```python
from build123d import *

# Parameters (mm, degrees)
SKETCH_1_W             = 140
SKETCH_1_H             = 60
EXTRUDE_1_DEPTH        = 5
SKETCH_2_R             = 1.2
CUT_EXTRUDE_1096_DEPTH = 153.397506541
SKETCH_4_R             = 1.4
CUT_EXTRUDE_3_DEPTH    = 5
PATTERN_LINEAR_1_COUNT = 3
PATTERN_LINEAR_1_PITCH = 40
SKETCH_6_R             = 2
CUT_EXTRUDE_4_DEPTH    = 1


with BuildPart() as part:
    # Sketch 1 → Extrude 1 (new body)
    with BuildSketch(Plane(origin=(0, 0, 0), x_dir=(1, 0, 0), z_dir=(0, 1, 0))):
        with Locations((70, -30)):
            Rectangle(SKETCH_1_W, SKETCH_1_H)
    extrude(amount=EXTRUDE_1_DEPTH)

    # Sketch 2 → Cut-Extrude 1096 (cut, through all)
    with BuildSketch(Plane(origin=(0, 5, 0), x_dir=(1, 0, 0), z_dir=(0, 1, 0))):
        with Locations(Location((102, -15, 0), (0, 0, 270))):
            Circle(SKETCH_2_R)
        with Locations(Location((118, -15, 0), (0, 0, 270))):
            Circle(SKETCH_2_R)
        with Locations(Location((102, -45, 0), (0, 0, 90))):
            Circle(SKETCH_2_R)
        with Locations(Location((118, -45, 0), (0, 0, 90))):
            Circle(SKETCH_2_R)
        with BuildLine():
            Line((100, -26.05), (100, -36.95))
            Line((100, -36.95), (104.2, -36.95))
            Line((104.2, -36.95), (104.2, -29.381860214))
            ThreePointArc((104.2, -29.381860214), (110, -31.5), (115.8, -29.381860214))
            Line((115.8, -29.381860214), (115.8, -36.95))
            Line((115.8, -36.95), (120, -36.95))
            Line((120, -36.95), (120, -26.05))
            Line((120, -26.05), (118.270278109, -26.05))
            ThreePointArc((118.270278109, -26.05), (110, -13.5), (101.729721891, -26.05))
            Line((101.729721891, -26.05), (100, -26.05))
        make_face()
    cut_extrude_1096 = extrude(amount=-CUT_EXTRUDE_1096_DEPTH, mode=Mode.SUBTRACT)

    # Sketch 4 → Cut-Extrude 3 (cut)
    with BuildSketch(Plane.ZY):
        with Locations((30, 2.5)):
            Circle(SKETCH_4_R)
        with Locations((8, 2.5)):
            Circle(SKETCH_4_R)
        with Locations((52, 2.5)):
            Circle(SKETCH_4_R)
    cut_extrude_3 = extrude(amount=-CUT_EXTRUDE_3_DEPTH, mode=Mode.SUBTRACT)

    # Mirror 1: Cut-Extrude 3 across plane
    add(cut_extrude_3.mirror(Plane(origin=(70, 0, 0), x_dir=(0, 0, 1), z_dir=(1, 0, 0))), mode=Mode.SUBTRACT)

    # Pattern Linear 1: Cut-Extrude 1096 ×3
    with Locations(*[(-i * PATTERN_LINEAR_1_PITCH, 0, 0) for i in range(1, PATTERN_LINEAR_1_COUNT)]):
        add(cut_extrude_1096, mode=Mode.SUBTRACT)

    # Sketch 6 → Cut-Extrude 4 (cut)
    with BuildSketch(Plane.XZ):
        with Locations(Location((22, 45, 0), (0, 0, 270))):
            Circle(SKETCH_6_R)
        with Locations(Location((38, 45, 0), (0, 0, 270))):
            Circle(SKETCH_6_R)
        with Locations(Location((62, 45, 0), (0, 0, 270))):
            Circle(SKETCH_6_R)
        with Locations(Location((78, 45, 0), (0, 0, 270))):
            Circle(SKETCH_6_R)
        with Locations(Location((102, 45, 0), (0, 0, 270))):
            Circle(SKETCH_6_R)
        with Locations(Location((118, 45, 0), (0, 0, 270))):
            Circle(SKETCH_6_R)
    extrude(amount=-CUT_EXTRUDE_4_DEPTH, mode=Mode.SUBTRACT)


solid = part.part
```
Verification items for the finished model (mm, model axes). A direction names the side the tool comes from. Coordinates: 2 decimals unless noted, no trailing zeros. Loops run counter-clockwise (first coordinate to the right, second up) from the corner with the lowest first, then second, coordinate; pieces in that order, holes last. Notation, with made-up numbers: (2.5, -2.5) -> (55.5, -2.5) arc R6 ccw to (55.5, 2.5) -> close; hole circle Ø3 at (56, 38). An arc over 180 degrees is marked (long way). Answer in a Markdown table with one row per item. Add a question column.
1. Depth check by flat-ended pin: P1, Ø3, axis at x = 62, z = 45, coming from the -Y side. Enter the tip coordinate at first touch or a pass-through.
2. Section check A-A, the plane x = 30. Enter the section's corners in (y, z), then the cut area to 3 significant figures.
3. Section check B-B, the plane z = 22.5. Enter the section's corners in (x, y).
4. Section check D-D, the plane y = 2.5. Give the number of separate pieces and of enclosed holes in the cut face, then the cut area to 3 significant figures.
5. Section check C-C, the plane z = 52. Enter the section's corners in (x, y).
6. Draft check along X on faces 4 (the face through (2.46, 1.65, 6.89)), 5 (the face through (21.234, 0.493, 43.153)), 6 (the face through (135, 3, 30)), 7 (the face through (117, 1, 44)). Enter one of: +X half, -X half, draft (parallel to the pull), parting line (faces both ways), or undercut.
7. Access from +Z, -Z, +X, -X, +Y, -Y to the whole of each face (thin tool, end or side, straight path). Record for faces 1 (the face through (80, 3, 32)), 2 (the face through (135, 3, 52)), 3 (the face through (2.46, 1.96, 53.29)).
8. Material ranges on probe 1 along X at (y, z) = (2.15, 27); probe 2 along X at (y, z) = (2.3, 22.5); probe 3 along Z at (x, y) = (77, 2.8), recorded low to high. Write a range as [from, to].
Derived:
| question | item | result |
|---|---|---|
| 1 | P1 | stops at y = 1 |
| 2 | outline | (0, 0) -> (5, 0) -> (5, 13.5) -> (0, 13.5) -> close; (0, 31.5) -> (5, 31.5) -> (5, 60) -> (0, 60) -> close |
| 2 | area | 210 mm² |
| 3 | outline | (0, 0) -> (21, 0) -> (21, 5) -> (0, 5) -> close; (39, 0) -> (61, 0) -> (61, 5) -> (39, 5) -> close; (79, 0) -> (101, 0) -> (101, 5) -> (79, 5) -> close; (119, 0) -> (140, 0) -> (140, 5) -> (119, 5) -> close |
| 4 | separate pieces | 1 |
| 4 | enclosed holes | 15 |
| 4 | area | 7,250 mm² |
| 5 | outline | (0, 0) -> (140, 0) -> (140, 1.1) -> (135, 1.1) -> (135, 3.9) -> (140, 3.9) -> (140, 5) -> (0, 5) -> (0, 3.9) -> (5, 3.9) -> (5, 1.1) -> (0, 1.1) -> close |
| 6 | face 4 | draft |
| 6 | face 5 | undercut |
| 6 | face 6 | +X half |
| 6 | face 7 | undercut |
| 7 | face 1 | +Y, -Y |
| 7 | face 2 | +X |
| 7 | face 3 | -X |
| 8 | probe 1 | x = [0, 20], [40, 60], [80, 100], [120, 140] |
| 8 | probe 2 | x = [0, 21], [39, 61], [79, 101], [119, 140] |
| 8 | probe 3 | z = [0, 14.34], [15.66, 16.84], [36.95, 44.34], [45.66, 60] |
